Answer from the drawing. Dimensions are ordinates in mm from the lowest x, y and z of the part. A direction names the side the tool comes from. Coordinates: 2 decimals unless noted, no trailing zeros. Loops run counter-clockwise (first coordinate to the right, second up) from the corner with the lowest first, then second, coordinate; pieces in that order, holes last. Notation, with made-up numbers: (75.25, -20.5) -> (93.25, -20.5) arc R10 cw to (93.25, -16.5) -> close; hole circle Ø3 at (-40, 38.25). An arc over 180 degrees is marked (long way). Answer as CSV lines item,"result".
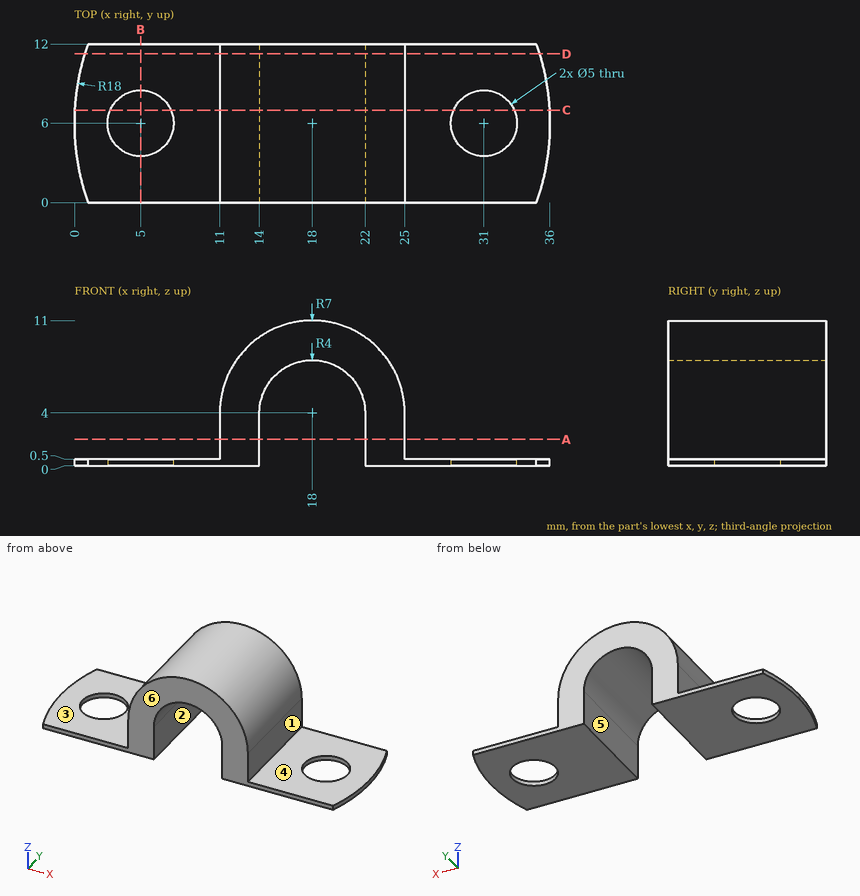
(1) For a pull along X with two mould halves and no side action, classify the marked faces 1, 2 and 3 as pulls with the +X half, pulls with the -X half, needs draft (parallel to the pull), parting line crosses it, or undercut.
Computed values:
face 1,"pulls with the +X half"
face 2,"undercut"
face 3,"needs draft"
(2) Flat-ended cylindrical pins translate along their axes: pin 1 Ø3 at (y, z) = (3.5, 1.5) entering from -X; pin 2 Ø1 at (x, y) = (26.5, 6) entering from +Z; pin 3 Ø4 at (y, z) = (3, 3) entering from -X; pin 4 Ø2 at (x, y) = (26, 4.5) entering from -Z. Find the tip coordinate at first contact, or state that the pin passes through.
Computed values:
pin 1,"x = 0.05"
pin 2,"z = 0.5"
pin 3,"x = 11"
pin 4,"z = 0"
(3) A cutting plane is placed at C-C, the plane y = 7. Write down the section's boundary in (x, z), and give its area (3 significant figures).
Computed values:
outline,"(0.03, 0) -> (2.71, 0) -> (2.71, 0.5) -> (0.03, 0.5) -> close; (7.29, 0) -> (14, 0) -> (14, 4) arc R4 cw to (22, 4) -> (22, 0) -> (28.71, 0) -> (28.71, 0.5) -> (25, 0.5) -> (25, 4) arc R7 ccw to (11, 4) -> (11, 0.5) -> (7.29, 0.5) -> close; (33.29, 0) -> (35.97, 0) -> (35.97, 0.5) -> (33.29, 0.5) -> close"
area,"82.2 mm2"
(4) Which of the six approach directions +Z, -Z, +X, -X, +Y, -Y give full straight-line access (tool end or side, diameter ignored) to the marked faces 4, 5 and 6?
Computed values:
face 4,"+Z, +X, +Y, -Y"
face 5,"-Z, +Y, -Y"
face 6,"+Z, -Z, +X, -X, -Y"
(5) A cutting plane is placed at B-B, the plane x = 5. Write down the section's boundary in (y, z), and give its area (3 significant figures).
Computed values:
outline,"(0, 0) -> (3.5, 0) -> (3.5, 0.5) -> (0, 0.5) -> close; (8.5, 0) -> (12, 0) -> (12, 0.5) -> (8.5, 0.5) -> close"
area,"3.50 mm2"
(6) Consider line 1 along Y through (x, z) = (5, 0.2); line 2 along X through (y, z) = (1, 4); line 3 along Z through (x, y) = (32.5, 3.75). Determine where each line is inside the solid, lowest interval first.
Computed values:
line 1,"0 to 3.5, 8.5 to 12"
line 2,"11 to 14, 22 to 25"
line 3,"0 to 0.5"
(7) A cutting plane is placed at D-D, the plane y = 11.25. Write down the section's boundary in (x, z).
Computed values:
outline,"(0.78, 0) -> (14, 0) -> (14, 4) arc R4 cw to (22, 4) -> (22, 0) -> (35.22, 0) -> (35.22, 0.5) -> (25, 0.5) -> (25, 4) arc R7 ccw to (11, 4) -> (11, 0.5) -> (0.78, 0.5) -> close"
(8) A cutting plane is placed at A-A, the plane z = 2. Write down the section's boundary in (x, y).
Computed values:
outline,"(11, 0) -> (14, 0) -> (14, 12) -> (11, 12) -> close; (22, 0) -> (25, 0) -> (25, 12) -> (22, 12) -> close"
